from build123d import *

# Parameters (mm, degrees)
SKETCH_1_W          = 240
SKETCH_1_H          = 160
EXTRUDE_1_DEPTH     = 120
SKETCH_2_W          = 159
SKETCH_2_H          = 158
SKETCH_2_W_2        = 78
SKETCH_2_H_2        = 119
CUT_EXTRUDE_1_DEPTH = 119
CUT_EXTRUDE_2_REACH = 242
SKETCH_3_W          = 80
SKETCH_3_H          = 64
FILLET_1_R          = 1
FILLET_2_R          = 3


with BuildPart() as part:
    # 草圖1 → 填料-伸長1 (new body)
    with BuildSketch(Plane(origin=(0, 0, 0), x_dir=(1, 0, 0), z_dir=(0, 1, 0))):
        Rectangle(SKETCH_1_W, SKETCH_1_H)
    extrude(amount=EXTRUDE_1_DEPTH)

    # 草圖2 → 除料-伸長1 (cut)
    with BuildSketch(Plane(origin=(0, 120, 0), x_dir=(1, 0, 0), z_dir=(0, 1, 0))):
        with Locations((-39.5, 0)):
            Rectangle(SKETCH_2_W, SKETCH_2_H)
        with Locations((80, -19.5)):
            Rectangle(SKETCH_2_W_2, SKETCH_2_H_2)
    extrude(amount=-CUT_EXTRUDE_1_DEPTH, mode=Mode.SUBTRACT)

    # 草圖3 → 除料-伸長2 (cut, up to next)
    with BuildSketch(Plane(origin=(120, 0, 0), x_dir=(0, 0, -1), z_dir=(1, 0, 0)), mode=Mode.PRIVATE) as cut_extrude_2_sk1:
        with Locations((0, 88)):
            Rectangle(SKETCH_3_W, SKETCH_3_H)
    cut_extrude_2_tool1 = extrude(cut_extrude_2_sk1.sketch, amount=-CUT_EXTRUDE_2_REACH, mode=Mode.PRIVATE) & part.part
    add(cut_extrude_2_tool1.solids().sort_by_distance((120, 88, 0))[0], mode=Mode.SUBTRACT)

    # 圓角1
    fillet_1_edges = [part.edges().sort_by_distance(p)[0] for p in [
        (120, 60, 80),
        (-120, 60, 80),
        (-120, 60, -80),
        (120, 60, -80),
    ]]
    fillet(fillet_1_edges, radius=FILLET_1_R)

    # 圓角2
    fillet_2_edges = [part.edges().sort_by_distance(p)[0] for p in [
        (40, 1, 0),
        (-39.5, 1, 79),
        (40, 60.5, 79),
        (-119, 1, 0),
        (-119, 60.5, 79),
        (-39.5, 1, -79),
        (-119, 60.5, -79),
        (119, 1, 19.5),
        (119, 28.5, -40),
        (80, 1, 79),
        (119, 60.5, 79),
        (41, 1, 19.5),
        (80, 1, -40),
    ]]
    fillet(fillet_2_edges, radius=FILLET_2_R)


solid = part.part
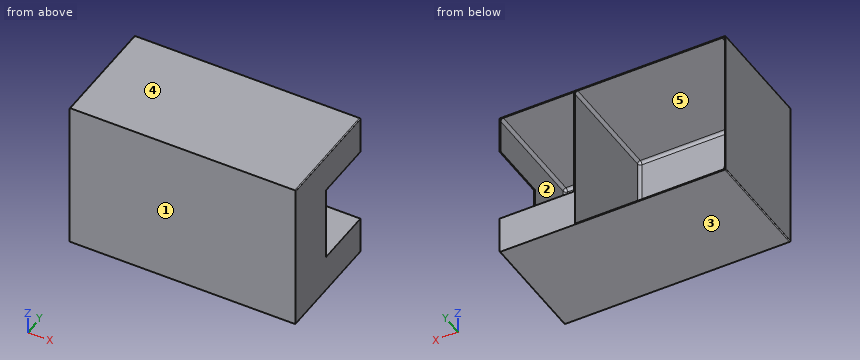
Geometry check sheet. Reference: the model listing, model coordinates, mm. Face numbers are marked on the shaded views. A direction names the side the tool comes from. Coordinates: 2 decimals unless noted, no trailing zeros. Order: outer loops, then holes, each group sorted by start corner. A loop starts at its lowest first (then second) coordinate and runs counter-clockwise, first axis right, second up. Notation, with made-up numbers: (78, 16) - (118, 16) arc R19 cw to (118, 34) - close; hole circle Ø11 at (52.5, 83.25). An arc over 180 degrees is marked (long way). One line per item, written item: value.
(1) Access from +Z, -Z, +X, -X, +Y, -Y to the whole of each face (thin tool, end or side, straight path). Record for the marked faces 4 and 5.
Data:
face 4: +Z, +X, -X, +Y, -Y
face 5: +Y
(2) Thickness scan on probe 1 along X at (y, z) = (23, -28); probe 2 along Z at (x, y) = (6, 105); probe 3 along Z at (x, y) = (78, 13.5). Record the ranges inside material, lowest first. Write a range as from..to.
Data:
probe 1: x = -120..-119, 40..41, 119..120
probe 2: z = -80..-79, 79..80
probe 3: z = -80..-40, 79..80
(3) Sectioned sample at C-C (y = 37.5). Enter the section's corners in (x, z), and give its area (3 significant figures).
Data:
outline: (-120, -79) arc R1 ccw to (-119, -80) - (119, -80) arc R1 ccw to (120, -79) - (120, 79) arc R1 ccw to (119, 80) - (-119, 80) arc R1 ccw to (-120, 79) - close; hole (-119, -76) arc R3 ccw to (-116, -79) - (40, -79) - (40, 76) arc R3 ccw to (37, 79) - (-116, 79) arc R3 ccw to (-119, 76) - close; hole (41, -40) - (116, -40) arc R3 ccw to (119, -37) - (119, 76) arc R3 ccw to (116, 79) - (41, 79) - close
area: 4,000 mm^2
(4) Release check for a two-part mould opening along Z. For the marked faces 1, 2 and 3 record: +Z half, -Z half, draft (parallel to the pull), parting line (faces both ways), or undercut.
Data:
face 1: draft
face 2: undercut
face 3: -Z half
(5) Sectioned sample at A-A (y = 102.5). Enter the section's corners in (x, z), and give its area (3 significant figures).
Data:
outline: (-120, -79) arc R1 ccw to (-119, -80) - (119, -80) arc R1 ccw to (120, -79) - (120, -40) - (41, -40) - (41, 79) - (116, 79) arc R3 cw to (119, 76) - (119, 40) - (120, 40) - (120, 79) arc R1 ccw to (119, 80) - (-119, 80) arc R1 ccw to (-120, 79) - close; hole (-119, -76) arc R3 ccw to (-116, -79) - (40, -79) - (40, 76) arc R3 ccw to (37, 79) - (-116, 79) arc R3 ccw to (-119, 76) - close
area: 3,920 mm^2
(6) Depth check by flat-ended pin: pin 1 Ø21.5 at (x, z) = (69, 9) entering from +Y; pin 2 Ø1.5 at (y, z) = (96.5, -26) entering from +X. Enter the tip coordinate at first touch or a pass-through.
Data:
pin 1: stops at y = 1
pin 2: stops at x = 41
(7) Sectioned sample at B-B (x = 89.5). Enter the section's corners in (y, z).
Data:
outline: (0, -80) - (120, -80) - (120, -40) - (4, -40) arc R3 cw to (1, -37) - (1, 76) arc R3 cw to (4, 79) - (120, 79) - (120, 80) - (0, 80) - close
(8) Sectioned sample at D-D (z = -61). Enter the section's corners in (x, y).
Data:
outline: (-120, 0) - (120, 0) - (120, 120) - (40, 120) - (40, 4) arc R3 cw to (37, 1) - (-116, 1) arc R3 cw to (-119, 4) - (-119, 120) - (-120, 120) - close
